Check sheet for the drawn part. Datum: minimum x, y, z corner. Units: mm. A direction names the side the tool comes from. Give positions to 0.01 mm unless a question says otherwise; leave off trailing zeros. Order: outer loops, then holes, each group sorted by start corner. A loop starts at its lowest first (then second) coordinate and runs counter-clockwise, first axis right, second up. Notation, with made-up numbers: (58, 54.25) - (104, 54.25) arc R32 ccw to (104, 92.25) - close; hole circle Ø10 at (78.25, -23.75). An arc over 180 degrees is marked (long way). Answer as a JSON object with one key per item and string values. Group by question number.
(1) Section check B-B (y = 15.5). Record the boundary of the cut face in (x, z), then the cut area to 3 significant figures.
(2) Mould release check, pull along X, two halves, no side actions. Record for the marked faces 1, 2 and 3: +X half, -X half, draft (parallel to the pull), parting line (faces both ways), or undercut.
(3) Thickness scan on line 1 (X direction, y = 31.5, z = 27); line 2 (X direction, y = 26.5, z = 30.5); line 3 (X direction, y = 4.5, z = 52). Record the ranges inside material, lowest first.
(4) Access from +Z, -Z, +X, -X, +Y, -Y to the whole of each face (thin tool, end or side, straight path). Record for the marked faces 4 and 5.
(5) Section check C-C (y = 26). Record the boundary of the cut face in (x, z).
(6) Depth check by flat-ended pin: pin 1 Ø2 at (x, y) = (82, 53.5) entering from +Z. Enter the tip coordinate at first touch or a pass-through.
(7) Section check D-D (x = 99). Record the boundary of the cut face in (y, z), then the cut area to 3 significant figures.
(8) Section check A-A (z = 23). Record the boundary of the cut face in (x, y).
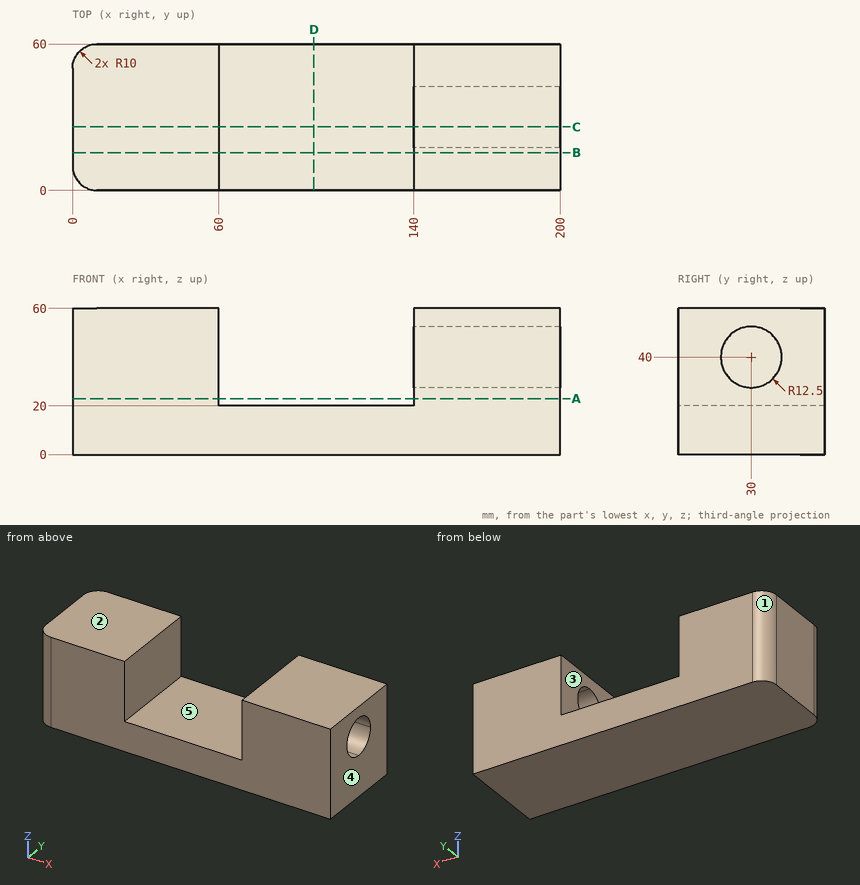
Solutions:
{
 "1": {"outline": "(0, 0) - (200, 0) - (200, 60) - (140, 60) - (140, 20) - (60, 20) - (60, 60) - (0, 60) - close", "area": "8,800 mm2"},
 "2": {"face 1": "-X half", "face 2": "draft", "face 3": "undercut"},
 "3": {"line 1": "x = 0 to 60, 140 to 200", "line 2": "x = 0 to 60", "line 3": "x = 1.65 to 60, 140 to 200"},
 "4": {"face 4": "+Z, -Z, +X, +Y, -Y", "face 5": "+Z, +Y, -Y"},
 "5": {"outline": "(0, 0) - (200, 0) - (200, 28.16) - (140, 28.16) - (140, 20) - (60, 20) - (60, 60) - (0, 60) - close; (140, 51.84) - (200, 51.84) - (200, 60) - (140, 60) - close"},
 "6": {"pin 1": "stops at z = 20"},
 "7": {"outline": "(0, 0) - (60, 0) - (60, 20) - (0, 20) - close", "area": "1,200 mm2"},
 "8": {"outline": "(0, 10) arc R10 ccw to (10, 0) - (60, 0) - (60, 60) - (10, 60) arc R10 ccw to (0, 50) - close; (140, 0) - (200, 0) - (200, 60) - (140, 60) - close"}
}
